```python
from build123d import *

# Parameters (mm, degrees)
F0_R     = 11
F1_DEPTH = 15
F2_R     = 16.15
F3_DEPTH = 38
F4_R     = 9.3
F5_DEPTH = 53.001
F7_R     = 11.7844294456
F8_DEPTH = 25


# Not quite as in the source:
# - a fillet or chamfer that OpenCascade refuses, or shapes differently, is made with other operations: its cross-section is extruded or revolved along the edge and cut away or added


with BuildPart() as f1:
    # F0 (on Top) → F1 (new body)
    with BuildSketch(Plane.XY):
        Circle(F0_R)
    extrude(amount=F1_DEPTH)

    # F2 (on face) → F3 (join)
    with BuildSketch(Plane.XY.offset(15)):
        Circle(F2_R)
    extrude(amount=F3_DEPTH)

    # F4 (on face) → F5 (cut, through all)
    with BuildSketch(Plane(origin=(0, 0, 0), x_dir=(1, 0, 0), z_dir=(0, 0, -1))):
        Circle(F4_R)
    extrude(amount=-F5_DEPTH, mode=Mode.SUBTRACT)

    # F7 (on offset) → F8 (cut)
    with BuildSketch(Plane.XY.offset(55)):
        Circle(F7_R)
    extrude(amount=-F8_DEPTH, mode=Mode.SUBTRACT)

    # F9: chamfer of 2 on 3 edges, made by hand

    # F9_s1 → F9_t2 (revolve, cut)
    with BuildSketch(Plane.XZ):
        Polygon((16.15, 51), (14.15, 53), (16.15, 53), align=None)
    revolve(axis=Axis((0, 0, 53), (0, 0, 1)), mode=Mode.SUBTRACT)

    # F9_s3 → F9_t4 (revolve, cut)
    with BuildSketch(Plane.XZ):
        Polygon((11, 2), (9, 0), (11, 0), align=None)
    revolve(axis=Axis((0, 0, 0), (0, 0, 1)), mode=Mode.SUBTRACT)

    # F9_s5 → F9_t6 (revolve, cut)
    with BuildSketch(Plane.XZ):
        Polygon((16.15, 17), (14.15, 15), (16.15, 15), align=None)
    revolve(axis=Axis((0, 0, 15), (0, 0, 1)), mode=Mode.SUBTRACT)


solid = f1.part
```
Source: CAD feature listing. Evaluate the final solid. Frame: model axes, mm. A direction names the side the tool comes from. Round coordinates to 2 decimals unless told otherwise and drop trailing zeros. Loops run counter-clockwise (first coordinate to the right, second up) from the corner with the lowest first, then second, coordinate; pieces in that order, holes last.
(1) Section query C-C (z = 27.5). Output: boundary loops of the cut face in (x, y).
From the geometry:
outline: circle Ø32.3 at (0, 0); hole circle Ø18.6 at (0, 0)
(2) Section query D-D (z = 13). Output: boundary loops of the cut face in (x, y), and give its area (3 significant figures).
From the geometry:
outline: circle Ø22 at (0, 0); hole circle Ø18.6 at (0, 0)
area: 108 mm2
(3) Access query for faces 1 (the cylindrical face through (-3.501, -15.766, 33.762)), 2 (the cylindrical face through (5.438, -10.455, 41.661)), 3 (the flat face through (-8.5, -7.3, 15)). Directions: +Z, -Z, +X, -X, +Y, -Y. A direction counts if a zero-diameter tool reaches every point of the face in a straight line with its end or side. Return the directions, or none.
From the geometry:
face 1: +Z, -Z
face 2: +Z
face 3: -Z
(4) Section query A-A (y = 0). Output: boundary loops of the cut face in (x, z).
From the geometry:
outline: (-16.15, 17) - (-14.15, 15) - (-11, 15) - (-11, 2) - (-9.3, 0.3) - (-9.3, 30) - (-11.78, 30) - (-11.78, 53) - (-14.15, 53) - (-16.15, 51) - close; (9.3, 0.3) - (11, 2) - (11, 15) - (14.15, 15) - (16.15, 17) - (16.15, 51) - (14.15, 53) - (11.78, 53) - (11.78, 30) - (9.3, 30) - close
(5) Material intervals for probe 1 along Y at (x, z) = (0, 10.5); probe 2 along Y at (x, z) = (0, 44.25); probe 3 along X at (y, z) = (2.5, 13), sorted ascending.
From the geometry:
probe 1: y = -11 to -9.3, 9.3 to 11
probe 2: y = -16.15 to -11.78, 11.78 to 16.15
probe 3: x = -10.71 to -8.96, 8.96 to 10.71
(6) Contact query for flat-ended pins moving along their axis: pin 1 Ø3 at (y, z) = (2, 23) entering from +X; pin 2 Ø1 at (x, z) = (-3.5, 7) entering from +Y; pin 3 Ø1.5 at (y, z) = (3, 46.5) entering from +X; pin 4 Ø12 at (x, z) = (5, 29.5) entering from -Y. Output: stop coordinate, or through.
From the geometry:
pin 1: stops at x = 16.14
pin 2: stops at y = 10.58
pin 3: stops at x = 15.99
pin 4: stops at y = -16.15
(7) Pull-direction query (X, two-part tool) for faces 4 (the flat face through (-5, 11, 53)), 5 (the flat face through (9, 4, 30)), 6 (the cylindrical face through (-2.38, -10.74, 8.41)); classes: +X half, -X half, draft (parallel to the pull), parting line (faces both ways), or undercut.
From the geometry:
face 4: draft
face 5: undercut
face 6: parting line
